from build123d import *

# Parameters (mm, degrees)
F0_W     = 2.9425137265
F0_H     = 28.5
F0_W_2   = 6
F0_H_2   = 14.5
F0_W_3   = 4
F0_H_3   = 68
F0_W_4   = 1
F1_DEPTH = 5
F0_R     = 1.5
F0_W_5   = 5
F0_H_4   = 5.2732650286
F0_H_5   = 7
F0_W_6   = 17.0574862735
F0_H_6   = 5.2732627955
F2_DEPTH = 8
F3_DEPTH = 15
F4_DEPTH = 10
F5_D     = 3


# Not quite as in the source:
# - a feature names something its author has since deleted; it is built from what else it names


with BuildPart() as f1:
    # F0 (on Top) → F1 (new body)
    with BuildSketch(Plane.XY):
        with Locations((-55.0466683022, -35.8276315331)):
            Rectangle(F0_W, F0_H)
        Polygon((-53.5754114389, -21.5776315331), (-53.5754114389, -50.0776315331), (-36.5179251655, -50.0776315331), (-36.5179251655, -12.0776315331), (-41.5179251655, -12.0776315331), (-41.5179251655, 17.9223684669), (-56.5179251655, 17.9223684669), (-56.5179251655, -21.5776315331), align=None)
        with Locations((-46.5179251655, -35.8276315331)):
            Rectangle(F0_W_2, F0_H_2, mode=Mode.SUBTRACT)
        Polygon((-36.5179251655, -12.0776315331), (-36.5179251655, -50.0776315331), (-31.5179251655, -50.0776315331), (-31.5179251655, 17.9223684669), (-36.5179251655, 17.9223684669), align=None)
        with Locations((-29.5179251655, -16.0776315331)):
            Rectangle(F0_W_3, F0_H_3)
        with Locations((-27.0179251655, -16.0776315331)):
            Rectangle(F0_W_4, F0_H_3)
        Polygon((-31.5179251655, 23.1956334954), (-31.5179251655, 17.9223684669), (-27.5179251655, 17.9223684669), (-26.5179251655, 17.9223684669), (-26.5179251655, 58.8525284669), (-2.0179251655, 58.8525284669), (-1.5179251655, 58.8525284669), (-1.0179251655, 58.8525284669), (23.4820748345, 58.8525284669), (23.4820748345, 17.9223684669), (24.4820748345, 17.9223684669), (28.4820748345, 17.9223684669), (28.4820748345, 23.1956312623), (28.4820748345, 64.1257884669), (-31.5179251655, 64.1257884669), align=None)
        Polygon((-26.5179251655, 17.9223684669), (-26.5179251655, -50.0776315331), (-2.0179251655, -50.0776315331), (-2.0179251655, 58.8525284669), (-26.5179251655, 58.8525284669), align=None)
        Polygon((-2.0179251655, 58.8525284669), (-2.0179251655, -50.0776315331), (-1.0179251655, -50.0776315331), (-1.0179251655, 58.8525284669), (-1.5179251655, 58.8525284669), align=None)
        Polygon((28.4820748345, 17.9223684669), (28.4820748345, -50.0776315331), (33.4820748345, -50.0776315331), (33.4820748345, -17.0776315331), (33.4820748345, -12.0776315331), (33.4820748345, 17.9223684669), align=None)
        with Locations((26.4820748345, -16.0776315331)):
            Rectangle(F0_W_3, F0_H_3)
        Polygon((-1.0179251655, 58.8525284669), (-1.0179251655, -50.0776315331), (23.4820748345, -50.0776315331), (23.4820748345, 17.9223684669), (23.4820748345, 58.8525284669), align=None)
        Polygon((33.4820748345, -17.0776315331), (33.4820748345, -50.0776315331), (53.4820748345, -50.0776315331), (53.4820748345, 17.9223684669), (38.4820748345, 17.9223684669), (38.4820748345, -12.0776315331), (33.4820748345, -12.0776315331), align=None)
        with Locations((23.9820748345, -16.0776315331)):
            Rectangle(F0_W_4, F0_H_3)
    extrude(amount=-F1_DEPTH)

    # F0 (on Top) → F2 (join)
    with BuildSketch(Plane.XY):
        Polygon((-27.5179251655, -50.0776315331), (-31.5179251655, -50.0776315331), (-31.5179251655, -57.0776315331), (28.4820748345, -57.0776315331), (28.4820748345, -50.0776315331), (24.4820748345, -50.0776315331), (23.4820748345, -50.0776315331), (-1.0179251655, -50.0776315331), (-2.0179251655, -50.0776315331), (-26.5179251655, -50.0776315331), align=None)
        Polygon((-56.5179251655, -57.0776315331), (-56.5179251655, -50.0776315331), (-56.5179251655, -21.5776315331), (-56.5179251655, 17.9223684669), (-41.5179251655, 17.9223684669), (-36.5179251655, 17.9223684669), (-36.5179251655, 23.1956334954), (-61.5179251655, 23.1956334954), (-61.5179251655, -57.0776315331), align=None)
        with Locations((-59.0179251655, -50.0776315331)):
            Circle(F0_R, mode=Mode.SUBTRACT)
        with Locations((-58.5054894246, 20.1860783767)):
            Circle(F0_R, mode=Mode.SUBTRACT)
        Polygon((33.4820748345, -50.0776315331), (33.4820748345, -57.0776315331), (58.4820748345, -57.0776315331), (58.4820748345, 23.1956312623), (33.4820748345, 23.1956312623), (33.4820748345, 17.9223684669), (38.4820748345, 17.9223684669), (53.4820748345, 17.9223684669), (53.4820748345, -50.0776315331), align=None)
        with Locations((55.9820748345, -50.0776315331)):
            Circle(F0_R, mode=Mode.SUBTRACT)
        with Locations((55.4806331986, 20.1810636766)):
            Circle(F0_R, mode=Mode.SUBTRACT)
        with Locations((-34.0179251655, 20.5590009811)):
            Rectangle(F0_W_5, F0_H_4)
        with Locations((-55.0466683022, -53.5776315331)):
            Rectangle(F0_W, F0_H_5)
        with Locations((-45.0466683022, -53.5776315331)):
            Rectangle(F0_W_6, F0_H_5)
        with Locations((-34.0179251655, -53.5776315331)):
            Rectangle(F0_W_5, F0_H_5)
        with Locations((30.9820748345, -53.5776315331)):
            Rectangle(F0_W_5, F0_H_5)
        with Locations((-27.0179251655, -16.0776315331)):
            Rectangle(F0_W_4, F0_H_3)
        with Locations((23.9820748345, -16.0776315331)):
            Rectangle(F0_W_4, F0_H_3)
        Polygon((-2.0179251655, 58.8525284669), (-2.0179251655, -50.0776315331), (-1.0179251655, -50.0776315331), (-1.0179251655, 58.8525284669), (-1.5179251655, 58.8525284669), align=None)
        with Locations((30.9820748345, 20.5589998646)):
            Rectangle(F0_W_5, F0_H_6)
        with Locations((-34.0179251655, 20.5590009811)):
            Rectangle(F0_W_5, F0_H_4)
        Polygon((-31.5179251655, 23.1956334954), (-31.5179251655, 17.9223684669), (-27.5179251655, 17.9223684669), (-26.5179251655, 17.9223684669), (-26.5179251655, 58.8525284669), (-2.0179251655, 58.8525284669), (-1.5179251655, 58.8525284669), (-1.0179251655, 58.8525284669), (23.4820748345, 58.8525284669), (23.4820748345, 17.9223684669), (24.4820748345, 17.9223684669), (28.4820748345, 17.9223684669), (28.4820748345, 23.1956312623), (28.4820748345, 64.1257884669), (-31.5179251655, 64.1257884669), align=None)
        with Locations((30.9820748345, 20.5589998646)):
            Rectangle(F0_W_5, F0_H_6)
        with Locations((-34.0179251655, 20.5590009811)):
            Rectangle(F0_W_5, F0_H_4)
    extrude(amount=-F2_DEPTH)

    # F0 (on Top) → F3 (join)
    with BuildSketch(Plane.XY):
        Polygon((-36.5179251655, -12.0776315331), (-36.5179251655, -50.0776315331), (-31.5179251655, -50.0776315331), (-31.5179251655, 17.9223684669), (-36.5179251655, 17.9223684669), align=None)
        with Locations((-34.0179251655, -53.5776315331)):
            Rectangle(F0_W_5, F0_H_5)
        with Locations((-34.0179251655, 20.5590009811)):
            Rectangle(F0_W_5, F0_H_4)
        with Locations((30.9820748345, -53.5776315331)):
            Rectangle(F0_W_5, F0_H_5)
        Polygon((28.4820748345, 17.9223684669), (28.4820748345, -50.0776315331), (33.4820748345, -50.0776315331), (33.4820748345, -17.0776315331), (33.4820748345, -12.0776315331), (33.4820748345, 17.9223684669), align=None)
        with Locations((30.9820748345, 20.5589998646)):
            Rectangle(F0_W_5, F0_H_6)
    extrude(amount=F3_DEPTH)

    # F0 (on Top) → F4 (join)
    with BuildSketch(Plane.XY):
        with Locations((-55.0466683022, -35.8276315331)):
            Rectangle(F0_W, F0_H)
        with Locations((-55.0466683022, -53.5776315331)):
            Rectangle(F0_W, F0_H_5)
    extrude(amount=F4_DEPTH)

    # F5 (through all)
    with Locations(Plane.XY):
        with Locations((35.9820748345, 20.5589998646), (35.9820748345, -14.5776315331), (-39.0179251655, 20.5589998646), (-39.0179251655, -14.5776315331)):
            Hole(F5_D / 2)


solid = f1.part
Can you work these out from the model? Positions are in its coordinate system, mm. A direction names the side the tool comes from. Give positions to 0.01 mm unless a question says otherwise; leave off trailing zeros. Order: outer loops, then holes, each group sorted by start corner. A loop starts at its lowest first (then second) coordinate and runs counter-clockwise, first axis right, second up. Notation, with made-up numbers: M 53,-2 L 100,-2 A36 ccw 100,34 Z; hole C 22,74 d10. An arc over 180 degrees is marked long. One line per item, written item: value.
Item 1: If we section it at B-B on x = -47: Write out the boundary of the cut face in (y, z), and give its area (3 significant figures).
Verdict:
outline: M -57.08,-8 L -50.08,-8 L -50.08,-5 L -43.08,-5 L -43.08,0 L -57.08,0 Z; M -28.58,-5 L 17.92,-5 L 17.92,-8 L 23.2,-8 L 23.2,0 L -28.58,0 Z
area: 366 mm2
Item 2: For pin 1 (4 mm diameter, centred on y = 51, z = -3.5, fed in from -X); pin 2 (12.5 mm diameter, centred on x = -9, y = 17.5, fed in from -Z); pin 3 (3.5 mm diameter, centred on x = 55.98, y = -50.08, fed in from +Z), each with a flat end and sliding along its axis, tell me the tip position at first contact or that it passes through.
Verdict:
pin 1: x = -31.52
pin 2: z = -5
pin 3: z = 0
Item 3: If we mould it in two halves opening along Y, with no side actions, what happens to faces 5 (the face through (-1.8, 3.8, -8)), 6 (the face through (11, -50.078, -6)), 7 (the face through (-41.518, 3, -2))? For each: pulls with the +Y half, pulls with the -Y half, needs draft (parallel to the pull), parting line crosses it, or undercut.
Verdict:
face 5: needs draft
face 6: undercut
face 7: undercut
Item 4: If we section it at D-D on z = 4.5: Write out the boundary of the cut face in (x, y).
Verdict:
outline: M -56.52,-57.08 L -53.58,-57.08 L -53.58,-21.58 L -56.52,-21.58 Z; M -36.52,-57.08 L -31.52,-57.08 L -31.52,23.2 L -36.52,23.2 Z; M 28.48,-57.08 L 33.48,-57.08 L 33.48,23.2 L 28.48,23.2 Z
Item 5: If we section it at C-C on y = 5.5: State how many separate pieces and enclosed holes the cut face has, and give its area (3 significant figures).
Verdict:
separate pieces: 3
enclosed holes: 0
area: 739 mm2
Item 6: For faces 1 (the face through (-42, -50.078, -6)), 2 (the face through (28.482, -16, 7)), 3 (the face through (46, -16, 0)), 4 (the face through (-43.518, -36, -2)), which set-ups out of +Z, -Z, +X, -X, +Y, -Y let a thin tool reach every point of the face, with its end or its side?
Verdict:
face 1: -Z
face 2: +Z, +Y, -Y
face 3: +Z, +X, +Y, -Y
face 4: +Z, -Z
Item 7: Please list where these lines run through material, in increasing order: line 1 (X direction, y = -4, z = -6); line 2 (X direction, y = 56, z = -6); line 3 (X direction, y = -38.5, z = 9.75).
Verdict:
line 1: -61.52 to -56.52, -27.52 to -26.52, -2.02 to -1.02, 23.48 to 24.48, 53.48 to 58.48
line 2: -31.52 to -26.52, -2.02 to -1.02, 23.48 to 28.48
line 3: -56.52 to -53.58, -36.52 to -31.52, 28.48 to 33.48
Item 8: If we section it at A-A on z = 13.5: Write out the boundary of the cut face in (x, y), and give its area (3 significant figures).
Verdict:
outline: M -36.52,-57.08 L -31.52,-57.08 L -31.52,23.2 L -36.52,23.2 Z; M 28.48,-57.08 L 33.48,-57.08 L 33.48,23.2 L 28.48,23.2 Z
area: 803 mm2
